The model under review builds one solid part; all positions refer to its coordinate system, in mm. A direction names the side the tool comes from. Coordinates: 2 decimals unless noted, no trailing zeros. Order: outer loops, then holes, each group sorted by start corner. A loop starts at its lowest first (then second) coordinate and runs counter-clockwise, first axis right, second up. Notation, with made-up numbers: (8.25, 41) -> (60.25, 41) arc R27 cw to (60.25, 59) -> close; hole circle Ø9 at (16.5, 38). An arc over 180 degrees is marked (long way). Use one line per item in the form item = value.
from build123d import *
from build123d.topology import SkipClean

# Parameters (mm, degrees)
SKETCH1_R               = 25.4
BASE_RING_DEPTH         = 12.7
SET_SCREW_R             = 2.413
SET_SCREW_HOLE_DEPTH    = 19.05
SET_SCREW_PATTERN_COUNT = 3
SET_SCREW_PATTERN_ANGLE = 180
UPPER_SECTION_DEPTH     = 21.59
LOWER_AXLE_D            = 5.1054
LOWER_AXLE_DEPTH        = 15.5575
LOWER_AXLE_CBORE_D      = 11.1125
LOWER_AXLE_CBORE_DEPTH  = 10.7442
UPPER_AXLE_D            = 5.1054
UPPER_AXLE_DEPTH        = 15.5575
UPPER_AXLE_CBORE_D      = 11.1125
UPPER_AXLE_CBORE_DEPTH  = 6.9342
SERVO_PLATE_SCREW_REACH = 51.66
SKETCH10_R              = 2.413
NUT_HOLE_DEPTH          = 2.54
LOWER_NUT_HOLE_DEPTH    = 2.54
FRONT_NUT_HOLE_DEPTH    = 2.54
FLUSH_PLATE_DEPTH       = 3.81
LEAD_IN_CHAMFER_SIZE    = 1.27


with BuildPart() as part:
    # Sketch1 → base_ring (new body)
    with BuildSketch(Plane(origin=(0, 0, 0), x_dir=(1, 0, 0), z_dir=(0, 1, 0))):
        with Locations(Location((0, 0, 0), (0, 0, 270))):
            Circle(SKETCH1_R)
        with BuildLine():
            Line((-1.905, 9.8425), (-20.632614806, 9.8425))
            ThreePointArc((-20.632614806, 9.8425), (-22.86, 0), (-20.632614806, -9.8425))
            Line((-20.632614806, -9.8425), (-1.905, -9.8425))
            Line((-1.905, -9.8425), (16.784650397, -9.8425))
            Line((16.784650397, -9.8425), (16.784650397, 9.8425))
            Line((16.784650397, 9.8425), (-1.905, 9.8425))
        make_face(mode=Mode.SUBTRACT)
    extrude(amount=BASE_RING_DEPTH)

    # set_screw → set_screw_hole (cut)
    with BuildSketch(Plane.XY.offset(25.4)):
        with Locations((0, 6.35)):
            Circle(SET_SCREW_R)
    set_screw_hole = extrude(amount=-SET_SCREW_HOLE_DEPTH, mode=Mode.SUBTRACT)

    # set_screw_pattern: set_screw_hole ×3 about axis
    set_screw_pattern_axis = Axis((0, 12.7, 0), (0, 1, 0))
    for i in range(1, SET_SCREW_PATTERN_COUNT):
        add(set_screw_hole.rotate(set_screw_pattern_axis, i * SET_SCREW_PATTERN_ANGLE / (SET_SCREW_PATTERN_COUNT - 1)), mode=Mode.SUBTRACT)

    # Sketch6 → upper_section (add)
    with BuildSketch(Plane(origin=(0, 12.7, 0), x_dir=(1, 0, 0), z_dir=(0, 1, 0))):
        with BuildLine():
            Line((-23.415490466, 9.8425), (-1.905, 9.8425))
            Line((-1.905, 9.8425), (-1.905, 17.4625))
            Line((-1.905, 17.4625), (14.752650397, 17.4625))
            ThreePointArc((14.752650397, 17.4625), (15.79854868, 16.522271624), (16.784650397, 15.519507435))
            Line((16.784650397, 15.519507435), (16.784650397, 9.8425))
            Line((16.784650397, 9.8425), (20.632614806, 9.8425))
            ThreePointArc((20.632614806, 9.8425), (22.86, 0), (20.632614806, -9.8425))
            Line((20.632614806, -9.8425), (16.784650397, -9.8425))
            Line((16.784650397, -9.8425), (16.784650397, -15.519507435))
            ThreePointArc((16.784650397, -15.519507435), (15.79854868, -16.522271624), (14.752650397, -17.4625))
            Line((14.752650397, -17.4625), (-1.905, -17.4625))
            Line((-1.905, -17.4625), (-1.905, -9.8425))
            Line((-1.905, -9.8425), (-23.415490466, -9.8425))
            ThreePointArc((-23.415490466, -9.8425), (25.4, 0), (-23.415490466, 9.8425))
        make_face()
    extrude(amount=UPPER_SECTION_DEPTH)

    # lower_axle
    with Locations(Plane.XY.offset(25.4)):
        with Locations((-12.7, 6.35)):
            lower_axle = CounterBoreHole(LOWER_AXLE_D / 2, LOWER_AXLE_CBORE_D / 2, LOWER_AXLE_CBORE_DEPTH, depth=LOWER_AXLE_DEPTH)

    # upper_axle
    with Locations(Plane.XY.offset(25.4)):
        with Locations((-6.35, 25.4)):
            upper_axle = CounterBoreHole(UPPER_AXLE_D / 2, UPPER_AXLE_CBORE_D / 2, UPPER_AXLE_CBORE_DEPTH, depth=UPPER_AXLE_DEPTH)

    # Sketch10 → servo_plate_screw (cut, up to next)
    with BuildSketch(Plane.XZ, mode=Mode.PRIVATE) as servo_plate_screw_sk1:
        with Locations(Location((8.89, 13.97, 0), (0, 0, 270))):
            Circle(SKETCH10_R)
    servo_plate_screw_tool1 = extrude(servo_plate_screw_sk1.sketch, amount=-SERVO_PLATE_SCREW_REACH, mode=Mode.PRIVATE) & part.part
    servo_plate_screw = servo_plate_screw_tool1.solids().sort_by_distance((8.89, 0, 13.97))[0]
    add(servo_plate_screw, mode=Mode.SUBTRACT)

    # Sketch11 → nut_hole (cut, symmetric)
    with BuildSketch(Plane(origin=(0, 12.7, 0), x_dir=(1, 0, 0), z_dir=(0, 1, 0))):
        Polygon((14.755878735, -13.97), (11.822939367, -8.89), (5.957060633, -8.89), (3.024121265, -13.97), (5.957060633, -19.05), (11.822939367, -19.05), align=None)
    nut_hole = extrude(amount=NUT_HOLE_DEPTH, both=True, mode=Mode.SUBTRACT)

    # Sketch12 → lower_nut_hole (cut)
    with BuildSketch(Plane(origin=(0, 0, 9.8425), x_dir=(-1, 0, 0), z_dir=(0, 0, -1))):
        Polygon((5.08, 3.417060633), (5.08, 9.282939367), (0, 12.215878735), (-5.08, 9.282939367), (-5.08, 3.417060633), (0, 0.484121265), align=None)
    lower_nut_hole = extrude(amount=-LOWER_NUT_HOLE_DEPTH, mode=Mode.SUBTRACT)

    # Sketch13 → front_nut_hole (cut)
    with BuildSketch(Plane.ZY.offset(-16.784650397)):
        Polygon((0, 12.215878735), (-5.08, 9.282939367), (-5.08, 3.417060633), (0, 0.484121265), (5.08, 3.417060633), (5.08, 9.282939367), align=None)
    extrude(amount=-FRONT_NUT_HOLE_DEPTH, mode=Mode.SUBTRACT)

    # screw_mirror: lower_axle, upper_axle, servo_plate_screw, nut_hole, lower_nut_hole across plane
    add(lower_axle.mirror(Plane.XY), mode=Mode.SUBTRACT)
    add(upper_axle.mirror(Plane.XY), mode=Mode.SUBTRACT)
    add(servo_plate_screw.mirror(Plane.XY), mode=Mode.SUBTRACT)
    add(nut_hole.mirror(Plane.XY), mode=Mode.SUBTRACT)
    add(lower_nut_hole.mirror(Plane.XY), mode=Mode.SUBTRACT)

    # Sketch9 → flush_plate (add)
    with SkipClean():  # the faces are left unmerged after this step: merging them gives an invalid solid
        with BuildSketch(Plane(origin=(0, 34.29, 0), x_dir=(1, 0, 0), z_dir=(0, 1, 0))):
            with BuildLine():
                Line((-18.445083186, 17.4625), (18.445083186, 17.4625))
                ThreePointArc((18.445083186, 17.4625), (0, 25.4), (-18.445083186, 17.4625))
            make_face()
            with BuildLine():
                Line((-18.445083186, -17.4625), (18.445083186, -17.4625))
                ThreePointArc((18.445083186, -17.4625), (0, -25.4), (-18.445083186, -17.4625))
            make_face()
        extrude(amount=FLUSH_PLATE_DEPTH)

    # lead_in_chamfer
    lead_in_chamfer_edges = [part.edges().sort_by_distance(p)[0] for p in [
        (0, 38.1, -17.4625),
        (0, 38.1, 17.4625),
        (-1.905, 34.29, -13.6525),
        (15.79854868, 34.29, -16.522271624),
        (16.784650397, 34.29, -12.681003718),
        (16.784650397, 34.29, 12.681003718),
        (15.79854868, 34.29, 16.522271624),
        (-1.905, 34.29, 13.6525),
    ]]
    chamfer(lead_in_chamfer_edges, length=LEAD_IN_CHAMFER_SIZE)


solid = part.part
Item 1: Tool access review of faces 4 (the face through (-1.05, 27.07, 21.21)), 5 (the face through (-13, 34.29, 14)), 6 (the face through (12.943, 12.171, -17.11)), 7 (the face through (17.411, 33.646, -12.969)): name each direction out of +Z, -Z, +X, -X, +Y, -Y from which nothing blocks a thin tool from reaching the whole face with its end or side.
Results found:
face_4 = +Z
face_5 = +X, -X, +Y
face_6 = none
face_7 = +Y
Item 2: Clearance check with flat-ended pins moving along their axes: pin 1 (7 mm diameter, centred on x = -7, y = 26.5, fed in from -Z); pin 2 (7.5 mm diameter, centred on x = 11, z = -12, fed in from +Y); pin 3 (2.5 mm diameter, centred on x = 21, z = -7.5, fed in from +Y). State where each tip first meets the part, or that it passes through.
Results found:
pin_1 = -18.47
pin_2 = 12.7
pin_3 = 34.29
Item 3: We need section C-C (y = 24). State how many separate pieces and enclosed holes the cut face has, plus the area to 3 significant figures.
Results found:
separate_pieces = 3
enclosed_holes = 0
area = 622 mm²
Item 4: We need section A-A (x = -19.5). Write out the cut boundary in (y, z).
Results found:
outline = (0, -16.28) -> (34.29, -16.28) -> (34.29, -9.84) -> (0, -9.84) -> close; (0, 9.84) -> (34.29, 9.84) -> (34.29, 16.28) -> (0, 16.28) -> close
Item 5: Draft analysis for pull direction Y (two halves, no side actions). For faces 1 (the face through (4.23, 11.45, 11.88)), 2 (the face through (-13, 34.29, -14)), 3 (the face through (-2.576, 10.729, -11.095)), state which applies: released by +Y, released by -Y, zero draft, split by the parting line, or undercut.
Results found:
face_1 = zero draft
face_2 = released by +Y
face_3 = undercut
Item 6: We need section D-D (x = 8.89). Write out the cut boundary in (y, z), plus the area to 3 significant figures.
Results found:
outline = (0, -23.79) -> (38.1, -23.79) -> (38.1, -18.73) -> (36.83, -17.46) -> (15.24, -17.46) -> (15.24, -19.05) -> (10.16, -19.05) -> (10.16, -16.38) -> (0, -16.38) -> close; (0, -11.56) -> (10.16, -11.56) -> (10.16, -9.84) -> (0, -9.84) -> close; (0, 9.84) -> (10.16, 9.84) -> (10.16, 11.56) -> (0, 11.56) -> close; (0, 16.38) -> (10.16, 16.38) -> (10.16, 19.05) -> (15.24, 19.05) -> (15.24, 17.46) -> (36.83, 17.46) -> (38.1, 18.73) -> (38.1, 23.79) -> (0, 23.79) -> close
area = 521 mm²
Item 7: To check wall thickness, follow L1, parallel to Y at x = 21.75, z = 0; L2, parallel to X at y = 8, z = 16; L3, parallel to Z at x = -17, y = 3. State the ranges of each line that lie inside material, in increasing order. Write a range as from..to.
Results found:
L1 = 0..3.94, 8.76..12.7
L2 = -19.73..-18.01, -7.39..-1.76, 1.76..7.59, 10.19..19.73
L3 = -14.66..-9.84, 9.84..14.66
Item 8: We need section B-B (z = -8.5). Write out the cut boundary in (x, y).
Results found:
outline = (-23.94, 0) -> (-21.22, 0) -> (-21.22, 12.7) -> (-23.94, 12.7) -> close; (16.78, 0) -> (23.94, 0) -> (23.94, 34.29) -> (21.22, 34.29) -> (21.22, 12.7) -> (16.78, 12.7) -> close
